```python
from build123d import *

# Parameters (mm, degrees)
SKETCH1_W               = 30
SKETCH1_H               = 80
BOSS_EXTRUDE1_DEPTH     = 10
SKETCH2_W               = 30
SKETCH2_H               = 13
BOSS_EXTRUDE2_DEPTH     = 81
CUT_EXTRUDE1_DEPTH      = 40
SKETCH4_W               = 20.2
SKETCH4_H               = 67
CUT_EXTRUDE2_DEPTH      = 5
SKETCH5_W               = 8
SKETCH5_H               = 2
CUT_EXTRUDE3_DEPTH      = 46
LPATTERN1_DEPTH         = 91
LPATTERN1_2_DEPTH       = 5
LPATTERN1_START         = 5
LPATTERN1_3_OUTLINE_W   = 9.8
LPATTERN1_3_OUTLINE_H   = 67
LPATTERN1_3_OUTLINE_W_2 = 4.9
LPATTERN1_3_DEPTH       = 5
LPATTERN1_START_2       = 10
LPATTERN1_4_DEPTH       = 41


# Read off the part's stored shape, not the designer's step: LPattern1
with BuildPart() as part:
    # Sketch1 → Boss-Extrude1 (new body)
    with BuildSketch(Plane(origin=(0, 0, 0), x_dir=(1, 0, 0), z_dir=(0, 1, 0))):
        Rectangle(SKETCH1_W, SKETCH1_H)
    extrude(amount=BOSS_EXTRUDE1_DEPTH)

    # Sketch2 → Boss-Extrude2 (add)
    with BuildSketch(Plane(origin=(0, 10, 0), x_dir=(1, 0, 0), z_dir=(0, 1, 0))):
        with Locations((0, -33.5)):
            Rectangle(SKETCH2_W, SKETCH2_H)
    extrude(amount=BOSS_EXTRUDE2_DEPTH)

    # Sketch3 → Cut-Extrude1 (cut)
    with BuildSketch(Plane(origin=(0, 91, 0), x_dir=(1, 0, 0), z_dir=(0, 1, 0))):
        Polygon((-4, -27), (4, -27), (4, -31), (7, -31), (4, -35), (-4, -35), (-7, -31), (-4, -31), align=None)
    extrude(amount=-CUT_EXTRUDE1_DEPTH, mode=Mode.SUBTRACT)

    # Sketch4 → Cut-Extrude2 (cut)
    with BuildSketch(Plane(origin=(0, 10, 0), x_dir=(1, 0, 0), z_dir=(0, 1, 0))):
        with Locations((0, 6.5)):
            Rectangle(SKETCH4_W, SKETCH4_H)
    extrude(amount=-CUT_EXTRUDE2_DEPTH, mode=Mode.SUBTRACT)

    # Sketch5 → Cut-Extrude3 (cut)
    with BuildSketch(Plane(origin=(0, 51, 0), x_dir=(1, 0, 0), z_dir=(0, 1, 0))):
        with Locations((0, -28)):
            Rectangle(SKETCH5_W, SKETCH5_H)
    extrude(amount=-CUT_EXTRUDE3_DEPTH, mode=Mode.SUBTRACT)

    # LPattern1 outline → LPattern1 (add)
    with BuildSketch(Plane(origin=(0, 0, 0), x_dir=(1, 0, 0), z_dir=(0, 1, 0))):
        Polygon((-34, -31), (-34, -27), (-56, -27), (-56, -31), (-53, -31), (-56, -35), (-64, -35), (-67, -31), (-64, -31), (-64, -27), (-75, -27), (-75, -40), (-15, -40), (-15, -27), (-26, -27), (-26, -31), (-23, -31), (-26, -35), (-34, -35), (-37, -31), align=None)
    extrude(amount=LPATTERN1_DEPTH)

    # LPattern1 2 outline → LPattern1 2 (add)
    with BuildSketch(Plane(origin=(0, 0, 0), x_dir=(1, 0, 0), z_dir=(0, 1, 0))):
        Polygon((-34, -27), (-34, -31), (-37, -31), (-34, -35), (-26, -35), (-23, -31), (-26, -31), (-26, -27), (-15, -27), (-15, 40), (-75, 40), (-75, -27), (-64, -27), (-64, -31), (-67, -31), (-64, -35), (-56, -35), (-53, -31), (-56, -31), (-56, -27), align=None)
    extrude(amount=LPATTERN1_2_DEPTH)

    # LPattern1 3 outline → LPattern1 3 (add)
    with BuildSketch(Plane(origin=(0, 0, 0), x_dir=(1, 0, 0), z_dir=(0, 1, 0)).offset(LPATTERN1_START)):
        with Locations((-45, 6.5)):
            Rectangle(LPATTERN1_3_OUTLINE_W, LPATTERN1_3_OUTLINE_H)
        Polygon((-26, -29), (-34, -29), (-34, -31), (-37, -31), (-34, -35), (-26, -35), (-23, -31), (-26, -31), align=None)
        with Locations((-17.45, 6.5)):
            Rectangle(LPATTERN1_3_OUTLINE_W_2, LPATTERN1_3_OUTLINE_H)
        Polygon((-56, -31), (-56, -29), (-64, -29), (-64, -31), (-67, -31), (-64, -35), (-56, -35), (-53, -31), align=None)
        with Locations((-72.55, 6.5)):
            Rectangle(LPATTERN1_3_OUTLINE_W_2, LPATTERN1_3_OUTLINE_H)
    extrude(amount=LPATTERN1_3_DEPTH)

    # LPattern1 4 outline → LPattern1 4 (add)
    with BuildSketch(Plane(origin=(0, 0, 0), x_dir=(1, 0, 0), z_dir=(0, 1, 0)).offset(LPATTERN1_START_2)):
        Polygon((-26, -29), (-34, -29), (-34, -31), (-37, -31), (-34, -35), (-26, -35), (-23, -31), (-26, -31), align=None)
        Polygon((-56, -31), (-56, -29), (-64, -29), (-64, -31), (-67, -31), (-64, -35), (-56, -35), (-53, -31), align=None)
    extrude(amount=LPATTERN1_4_DEPTH)


solid = part.part
```
Check sheet for the modelled part. Datum: model origin and axes. Units: mm. A direction names the side the tool comes from. Coordinates: 2 decimals unless noted, no trailing zeros. Write each loop counter-clockwise with the first axis right and the second up, starting at its lowest first coordinate (ties: lowest second). Pieces come first, ordered by that corner, then holes. Notation, with made-up numbers: M 61,56 L 95,56 A28 cw 95,85 Z; hole C 52.25,84.5 d6. An arc over 180 degrees is marked long. Use one line per item in the form item = value.
Item 1: Sectioned sample at A-A, the plane y = 38.5. Record the cut outline in (x, z), and give its area (3 significant figures).
Answer below:
outline = M -75,27 L -64,27 L -64,29 L -56,29 L -56,27 L -34,27 L -34,29 L -26,29 L -26,27 L -4,27 L -4,29 L 4,29 L 4,27 L 15,27 L 15,40 L -75,40 Z
area = 1,120 mm^2
Item 2: Material ranges on L1, parallel to X at y = 8.5, z = -32; L2, parallel to Z at x = -28, y = 81; L3, parallel to Z at x = 3.5, y = 25, recorded low to high. Write a range as from..to.
Answer below:
L1 = -75..-70.1, -49.9..-40.1, -19.9..-10.1, 10.1..15
L2 = 35..40
L3 = 29..40
Item 3: Sectioned sample at D-D, the plane y = 59.5. Record the cut outline in (x, z).
Answer below:
outline = M -75,27 L -64,27 L -64,31 L -67,31 L -64,35 L -56,35 L -53,31 L -56,31 L -56,27 L -34,27 L -34,31 L -37,31 L -34,35 L -26,35 L -23,31 L -26,31 L -26,27 L -4,27 L -4,31 L -7,31 L -4,35 L 4,35 L 7,31 L 4,31 L 4,27 L 15,27 L 15,40 L -75,40 Z
Item 4: Release check for a two-part mould opening along X. For faces 1 (the face through (-30, 5, -6)), 2 (the face through (-75, 28, 29)), 3 (the face through (-31, 91, 36)) record: pulls with the +X half, pulls with the -X half, needs draft (parallel to the pull), parting line crosses it, or undercut.
Answer below:
face_1 = undercut
face_2 = pulls with the -X half
face_3 = needs draft
Item 5: Sectioned sample at C-C, the plane z = -19. Record the cut outline in (x, y), and give its area (3 significant figures).
Answer below:
outline = M -75,0 L 15,0 L 15,10 L 10.1,10 L 10.1,5 L -10.1,5 L -10.1,10 L -19.9,10 L -19.9,5 L -40.1,5 L -40.1,10 L -49.9,10 L -49.9,5 L -70.1,5 L -70.1,10 L -75,10 Z
area = 597 mm^2
Item 6: Gauge pin test, flat ends, axial feed: pin 1 Ø4 at (x, y) = (-59, 67.5) entering from -Z; pin 2 Ø9 at (x, y) = (-29, 68) entering from -Z; pin 3 Ø3 at (x, z) = (-39.5, 5.5) entering from -Y; pin 4 Ø22 at (x, z) = (-28, -9.5) entering from +Y. Record the tip position at first contact, or that the pin passes through.
Answer below:
pin_1 = 35
pin_2 = 27
pin_3 = 0
pin_4 = 10
Item 7: Sectioned sample at B-B, the plane x = -0.5. Record the cut outline in (y, z).
Answer below:
outline = M 0,-40 L 5,-40 L 5,29 L 51,29 L 51,35 L 91,35 L 91,40 L 0,40 Z
Item 8: Set-up check for faces 4 (the face through (-45, 10, -7)), 5 (the face through (0, 71, 35)): record each of +Z, -Z, +X, -X, +Y, -Y from which the full face is reachable in a straight line by a thin tool's end or side.
Answer below:
face_4 = -Z, +X, -X, +Y
face_5 = -Z, +Y
